CAD build for the part. Positions are in the model's coordinates, mm. Face numbers are marked on the shaded views. A direction names the side the tool comes from. Round coordinates to 2 decimals unless told otherwise and drop trailing zeros. Loops run counter-clockwise (first coordinate to the right, second up) from the corner with the lowest first, then second, coordinate; pieces in that order, holes last. Notation, with made-up numbers: M 6,-3 L 32,-3 A23 cw 32,34 Z; hole C 65.5,-3 d11. An arc over 180 degrees is marked long. One line per item, written item: value. Start each with the question number.
from build123d import *

# Parameters (mm, degrees)
SKETCH1_W                                       = 5
SKETCH1_H                                       = 25
SKETCH1_W_2                                     = 110
SKETCH1_H_2                                     = 5
SKETCH1_W_3                                     = 290
BOSS_EXTRUDE1_DEPTH                             = 120
SKETCH2_W                                       = 90
SKETCH2_H                                       = 65
SKETCH2_R                                       = 5
CUT_EXTRUDE1_DEPTH                              = 320.452656899
CSK_FOR_M2_FLAT_HEAD_MACHINE_SCREW1_D           = 2.4
CSK_FOR_M2_FLAT_HEAD_MACHINE_SCREW1_CSINK_D     = 4.4
CSK_FOR_M2_FLAT_HEAD_MACHINE_SCREW1_CSINK_ANGLE = 90
F_3_0MM_DOWEL_HOLE1_D                           = 3
BOSS_EXTRUDE2_DEPTH                             = 120
SKETCH10_W                                      = 36.666666667
SKETCH10_H                                      = 20
SKETCH10_W_2                                    = 36.666666666
CUT_EXTRUDE2_DEPTH                              = 290
FILLET1_R                                       = 5
CSK_FOR_M3_FLAT_HEAD_MACHINE_SCREW1_D           = 3.4
CSK_FOR_M3_FLAT_HEAD_MACHINE_SCREW1_DEPTH       = 5
CSK_FOR_M3_FLAT_HEAD_MACHINE_SCREW1_CSINK_D     = 6.3
CSK_FOR_M3_FLAT_HEAD_MACHINE_SCREW1_CSINK_ANGLE = 90
CSK_FOR_M3_FLAT_HEAD_MACHINE_SCREW1_TIP         = 1.021463052
FILLET2_R                                       = 2


with BuildPart() as part:
    # Sketch1 → Boss-Extrude1 (new body)
    with BuildSketch(Plane(origin=(0, 0, 0), x_dir=(0, 0, -1), z_dir=(1, 0, 0))):
        with Locations((-2.5, 12.5)):
            Rectangle(SKETCH1_W, SKETCH1_H)
        with Locations((55, 2.5)):
            Rectangle(SKETCH1_W_2, SKETCH1_H_2)
        with Locations((-150, 22.5)):
            Rectangle(SKETCH1_W_3, SKETCH1_H_2)
    extrude(amount=BOSS_EXTRUDE1_DEPTH)

    # Sketch2 → Cut-Extrude1 (cut, through all)
    with BuildSketch(Plane(origin=(0, 25, 0), x_dir=(1, 0, 0), z_dir=(0, 1, 0))):
        with BuildLine():
            Line((34, -272), (34, -270.101020514))
            ThreePointArc((34, -270.101020514), (31.464466094, -271.464466094), (30.101020514, -274))
            Line((30.101020514, -274), (32, -274))
            Line((32, -274), (32, -276))
            Line((32, -276), (30.101020514, -276))
            ThreePointArc((30.101020514, -276), (31.464466094, -278.535533906), (34, -279.898979486))
            Line((34, -279.898979486), (34, -278))
            Line((34, -278), (36, -278))
            Line((36, -278), (36, -279.898979486))
            ThreePointArc((36, -279.898979486), (38.535533906, -278.535533906), (39.898979486, -276))
            Line((39.898979486, -276), (38, -276))
            Line((38, -276), (38, -274))
            Line((38, -274), (39.898979486, -274))
            ThreePointArc((39.898979486, -274), (38.535533906, -271.464466094), (36, -270.101020514))
            Line((36, -270.101020514), (36, -272))
            Line((36, -272), (34, -272))
        make_face()
        with BuildLine():
            Line((84, -272), (84, -270.101020514))
            ThreePointArc((84, -270.101020514), (81.464466094, -271.464466094), (80.101020514, -274))
            Line((80.101020514, -274), (82, -274))
            Line((82, -274), (82, -276))
            Line((82, -276), (80.101020514, -276))
            ThreePointArc((80.101020514, -276), (81.464466094, -278.535533906), (84, -279.898979486))
            Line((84, -279.898979486), (84, -278))
            Line((84, -278), (86, -278))
            Line((86, -278), (86, -279.898979486))
            ThreePointArc((86, -279.898979486), (88.535533906, -278.535533906), (89.898979486, -276))
            Line((89.898979486, -276), (88, -276))
            Line((88, -276), (88, -274))
            Line((88, -274), (89.898979486, -274))
            ThreePointArc((89.898979486, -274), (88.535533906, -271.464466094), (86, -270.101020514))
            Line((86, -270.101020514), (86, -272))
            Line((86, -272), (84, -272))
        make_face()
        with Locations((60, 32.5)):
            Rectangle(SKETCH2_W, SKETCH2_H)
        with BuildLine():
            Line((-14.667196701, 131.62219227), (15, 110))
            add(Edge.make_bspline(
                [(15, 110), (0, 110), (0, 65)],
                knots=[0, 0, 0, 1.570796327, 1.570796327, 1.570796327], degree=2, weights=[1, 0.707106781, 1]))
            Line((0, 65), (-14.667196701, 131.62219227))
        make_face()
        with BuildLine():
            add(Edge.make_bspline(
                [(120, 65), (120, 110), (105, 110)],
                knots=[4.71238898, 4.71238898, 4.71238898, 6.283185307, 6.283185307, 6.283185307], degree=2, weights=[1, 0.707106781, 1]))
            Line((105, 110), (141.916619914, 126.007078186))
            Line((141.916619914, 126.007078186), (120, 65))
        make_face()
        with Locations(Location((60, -35, 0), (0, 0, 270))):
            Circle(SKETCH2_R)
        with Locations(Location((60, -85, 0), (0, 0, 270))):
            Circle(SKETCH2_R)
    extrude(amount=-CUT_EXTRUDE1_DEPTH, mode=Mode.SUBTRACT)

    # CSK for M2 Flat Head Machine Screw1 (through all)
    with Locations(Plane(origin=(0, 5, 0), x_dir=(1, 0, 0), z_dir=(0, 1, 0))):
        with Locations((40, 102.5), (80, 102.5)):
            CounterSinkHole(CSK_FOR_M2_FLAT_HEAD_MACHINE_SCREW1_D / 2, CSK_FOR_M2_FLAT_HEAD_MACHINE_SCREW1_CSINK_D / 2, counter_sink_angle=CSK_FOR_M2_FLAT_HEAD_MACHINE_SCREW1_CSINK_ANGLE)

    # Ø3.0mm Dowel Hole1 (through all)
    with Locations(Plane(origin=(0, 25, 0), x_dir=(1, 0, 0), z_dir=(0, 1, 0))):
        with Locations((23.25, -75.11), (32.5, -81.11), (41.75, -75.11)):
            Hole(F_3_0MM_DOWEL_HOLE1_D / 2)

    # Sketch9 → Boss-Extrude2 (add)
    with BuildSketch(Plane.ZY):
        Polygon((5, 0), (25, 20), (5, 20), align=None)
    extrude(amount=-BOSS_EXTRUDE2_DEPTH)

    # Sketch10 → Cut-Extrude2 (cut)
    with BuildSketch(Plane.XY.offset(295)):
        with Locations((18.333333334, 10)):
            Rectangle(SKETCH10_W, SKETCH10_H)
        with Locations((60, 10)):
            Rectangle(SKETCH10_W_2, SKETCH10_H)
        with Locations((101.666666667, 10)):
            Rectangle(SKETCH10_W, SKETCH10_H)
    extrude(amount=-CUT_EXTRUDE2_DEPTH, mode=Mode.SUBTRACT)

    # Fillet1
    fillet1_edges = [part.edges().sort_by_distance(p)[0] for p in [
        (60, 25, 0),
        (18.333333333, 20, 5),
        (60, 20, 5),
        (101.666666667, 20, 5),
    ]]
    fillet(fillet1_edges, radius=FILLET1_R)

    # CSK for M3 Flat Head Machine Screw1
    with Locations(Plane.XZ):
        with Locations((25, -70)):
            CounterSinkHole(CSK_FOR_M3_FLAT_HEAD_MACHINE_SCREW1_D / 2, CSK_FOR_M3_FLAT_HEAD_MACHINE_SCREW1_CSINK_D / 2, depth=CSK_FOR_M3_FLAT_HEAD_MACHINE_SCREW1_DEPTH, counter_sink_angle=CSK_FOR_M3_FLAT_HEAD_MACHINE_SCREW1_CSINK_ANGLE)
            with Locations((0, 0, -(CSK_FOR_M3_FLAT_HEAD_MACHINE_SCREW1_DEPTH + CSK_FOR_M3_FLAT_HEAD_MACHINE_SCREW1_TIP / 2))):  # 118° drill point
                Cone(0, CSK_FOR_M3_FLAT_HEAD_MACHINE_SCREW1_D / 2, CSK_FOR_M3_FLAT_HEAD_MACHINE_SCREW1_TIP, mode=Mode.SUBTRACT)

    # Fillet2
    fillet2_edges = [part.edges().sort_by_distance(p)[0] for p in [
        (60, 20, 80),
        (60, 25, 80),
    ]]
    fillet(fillet2_edges, radius=FILLET2_R)


solid = part.part
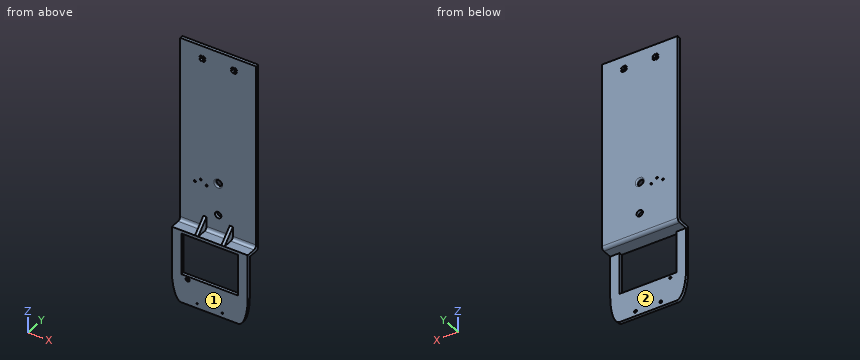
(1) Probe L1, parallel to X at y = 21.3, z = 75.11; L2, parallel to X at y = 2.05, z = -102.5; L3, parallel to X at y = 10.25, z = 6. List the from-to ranges inside material, lowest first.
(2) Slice it at A-A, the plane x = 48.5. List the corners of the cut face in (y, z).
(3) Flat gauge pins, fed straight in: P1, Ø1.5, axis at x = 88, y = 18, coming from the -Z side; P2, Ø0.6, axis at x = 39, y = 22.5, coming from the -Z side; P3, Ø2, axis at x = 80, z = -102.5, coming from the +Y side; P4, Ø10, axis at x = 74, z = 189.5, coming from the -Y side. Where does each tip first touch, or does it go through?
(4) Slice it at C-C, the plane z = 231.5. List the corners of the cut face in (x, y).
(5) Which spindle directions (+Z, -Z, +X, -X, +Y, -Y) get a long thin tool onto all of the face, cutting with end or side? Do the marked faces 1 and 2. Say none if no direction does.
(6) Slice it at B-B, the plane y = 9.75. List the corners of the cut face in (x, z), and give its area (4 significant figures).
Check result:
1. L1: x = 0 to 21.75, 24.75 to 40.25, 43.25 to 120
1. L2: x = 6.71 to 38.8, 41.2 to 78.8, 81.2 to 113.29
1. L3: x = 36.67 to 41.67, 78.33 to 83.33
2. outline: M 0,-110 L 5,-110 L 5,-65 L 0,-65 Z; M 0,0 L 20,0 A5 ccw 25,5 L 25,295 L 20,295 L 20,10 A5 cw 15,5 L 0,5 Z
3. P1: stops at z = 0
3. P2: stops at z = 0.51
3. P3: passes through
3. P4: stops at y = 20
4. outline: M 0,20 L 120,20 L 120,25 L 0,25 Z
5. face 1: +Z, -Z, +X, -X, -Y
5. face 2: -Z, +X, -X, +Y
6. outline: M 0,0 L 120,0 L 120,5 L 83.33,5 L 83.33,14.75 L 78.33,14.75 L 78.33,5 L 41.67,5 L 41.67,14.75 L 36.67,14.75 L 36.67,5 L 0,5 Z
6. area: 697.5 mm^2
